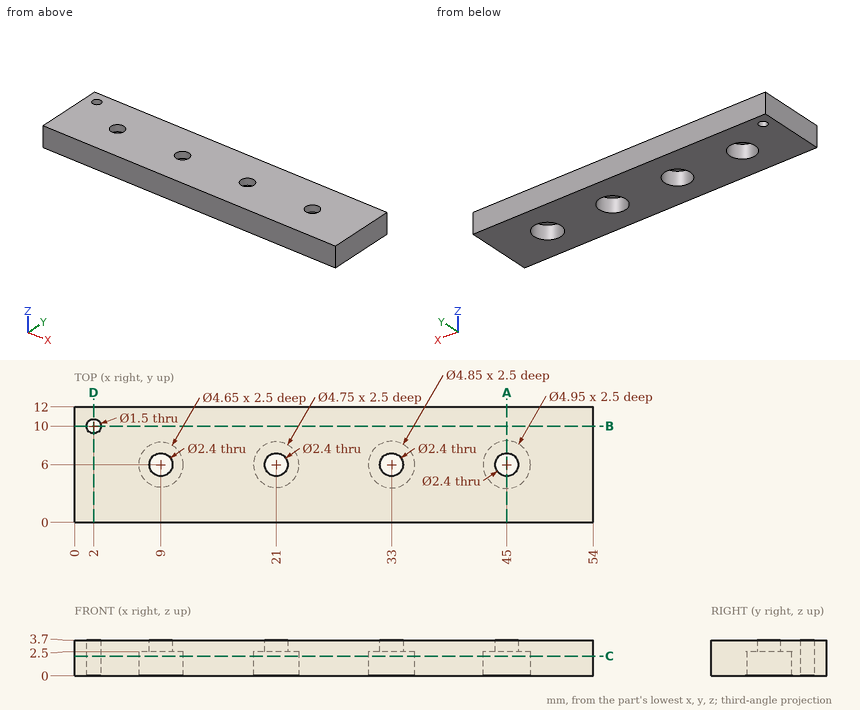
Drawing for the job (mm, zero at the part's lowest x, y, z). Give positions to 0.01 mm unless a question says otherwise; leave off trailing zeros. Loops run counter-clockwise (first coordinate to the right, second up) from the corner with the lowest first, then second, coordinate; pieces in that order, holes last.
Item 1: Slice it at B-B (y = 10). Write the cut outline in (x, z).
Check values:
outline: (0, 0) - (1.25, 0) - (1.25, 3.7) - (0, 3.7) - close; (2.75, 0) - (54, 0) - (54, 3.7) - (2.75, 3.7) - close
Item 2: Drill centre lines: line 1 along Y through (x, z) = (45, 2.8); line 2 along X through (y, z) = (6.75, 0.2); line 3 along Y through (x, z) = (45, 1.1) (3 decimals). Where is each one in solid material? Low to high.
Check values:
line 1: y = 0 to 4.8, 7.2 to 12
line 2: x = 0 to 6.8, 11.2 to 18.75, 23.25 to 30.69, 35.31 to 42.64, 47.36 to 54
line 3: y = 0 to 3.525, 8.475 to 12
Item 3: Slice it at A-A (x = 45). Write the cut outline in (y, z) (3 decimals), plus the area to 3 significant figures.
Check values:
outline: (0, 0) - (3.525, 0) - (3.525, 2.5) - (4.8, 2.5) - (4.8, 3.7) - (0, 3.7) - close; (7.2, 2.5) - (8.475, 2.5) - (8.475, 0) - (12, 0) - (12, 3.7) - (7.2, 3.7) - close
area: 29.1 mm2
Item 4: Slice it at C-C (z = 2.05). Write the cut outline in (x, y) (3 decimals), plus the area to 3 significant figures.
Check values:
outline: (0, 0) - (54, 0) - (54, 12) - (0, 12) - close; hole circle Ø1.5 at (2, 10); hole circle Ø4.65 at (9, 6); hole circle Ø4.75 at (21, 6); hole circle Ø4.85 at (33, 6); hole circle Ø4.95 at (45, 6)
area: 574 mm2
Item 5: Drop flat-ended pins along their axis: P1, Ø5.5, axis at x = 32.5, y = 5, coming from the -Z side; P2, Ø1.4, axis at x = 22, y = 6.5, coming from the -Z side. Give the stop position or say it passes through.
Check values:
P1: stops at z = 0
P2: stops at z = 2.5
Item 6: Slice it at D-D (x = 2). Write the cut outline in (y, z), plus the area to 4 significant figures.
Check values:
outline: (0, 0) - (9.25, 0) - (9.25, 3.7) - (0, 3.7) - close; (10.75, 0) - (12, 0) - (12, 3.7) - (10.75, 3.7) - close
area: 38.85 mm2
